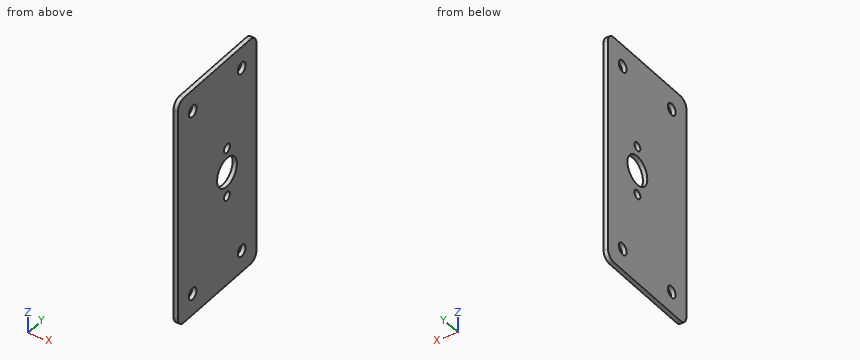
```python
from build123d import *

# Parameters (mm, degrees)
SKETCH_1_W      = 80
SKETCH_1_H      = 40
SKETCH_1_R      = 2
SKETCH_1_R_2    = 5.05
SKETCH_1_R_3    = 1.5
EXTRUDE_1_DEPTH = 1.5
FILLET_1_R      = 3


with BuildPart() as part:
    # ｽｹｯﾁ1 → ﾎﾞｽ - 押し出し1 (new body)
    with BuildSketch(Plane(origin=(0, 0, 0), x_dir=(0, 0, -1), z_dir=(1, 0, 0))):
        Rectangle(SKETCH_1_W, SKETCH_1_H)
        with Locations((32.5, 12.5)):
            Circle(SKETCH_1_R, mode=Mode.SUBTRACT)
        with Locations(Location((-32.5, 12.5, 0), (0, 0, 180))):
            Circle(SKETCH_1_R, mode=Mode.SUBTRACT)
        with Locations((32.5, -12.5)):
            Circle(SKETCH_1_R, mode=Mode.SUBTRACT)
        with Locations((0, 5)):
            Circle(SKETCH_1_R_2, mode=Mode.SUBTRACT)
        with Locations(Location((-32.5, -12.5, 0), (0, 0, 180))):
            Circle(SKETCH_1_R, mode=Mode.SUBTRACT)
        with Locations((8.5, 5)):
            Circle(SKETCH_1_R_3, mode=Mode.SUBTRACT)
        with Locations(Location((-8.5, 5, 0), (0, 0, 180))):
            Circle(SKETCH_1_R_3, mode=Mode.SUBTRACT)
    extrude(amount=EXTRUDE_1_DEPTH)

    # ﾌｨﾚｯﾄ1
    fillet_1_edges = [part.edges().sort_by_distance(p)[0] for p in [
        (0.75, -20, -40),
        (0.75, -20, 40),
        (0.75, 20, 40),
        (0.75, 20, -40),
    ]]
    fillet(fillet_1_edges, radius=FILLET_1_R)


solid = part.part
```
Could you check a few things on this model? Use its own coordinates, in mm. Give positions to 0.01 mm unless a question says otherwise; leave off trailing zeros. Loops run counter-clockwise (first coordinate to the right, second up) from the corner with the lowest first, then second, coordinate; pieces in that order, holes last. Notation, with made-up numbers: (-7, 26.5) -> (13, 26.5) arc R30 cw to (13, 65.5) -> close; hole circle Ø8 at (16, -18.75). An arc over 180 degrees is marked (long way). Put each result on its own line as item: value.
(1) Imagine slicing it at C-C on y = 5. Write out the boundary of the cut face in (x, z).
Computed:
outline: (0, -40) -> (1.5, -40) -> (1.5, -10) -> (0, -10) -> close; (0, -7) -> (1.5, -7) -> (1.5, -5.05) -> (0, -5.05) -> close; (0, 5.05) -> (1.5, 5.05) -> (1.5, 7) -> (0, 7) -> close; (0, 10) -> (1.5, 10) -> (1.5, 40) -> (0, 40) -> close
(2) Please list where these lines run through material, in increasing order: probe 1 along Y at (x, z) = (0.65, -32.5); probe 2 along Y at (x, z) = (0.3, -33.5); probe 3 along Z at (x, y) = (0.9, 11.5). Write a range as [from, to].
Computed:
probe 1: [-20, -14.5], [-10.5, 10.5], [14.5, 20]
probe 2: [-20, -14.23], [-10.77, 10.77], [14.23, 20]
probe 3: [-40, -34.23], [-30.77, 30.77], [34.23, 40]
(3) Imagine slicing it at A-A on z = 8.5. Write out the boundary of the cut face in (x, y).
Computed:
outline: (0, -20) -> (1.5, -20) -> (1.5, 3.5) -> (0, 3.5) -> close; (0, 6.5) -> (1.5, 6.5) -> (1.5, 20) -> (0, 20) -> close
(4) Imagine slicing it at B-B on z = 32.5. Write out the boundary of the cut face in (x, y).
Computed:
outline: (0, -20) -> (1.5, -20) -> (1.5, -14.5) -> (0, -14.5) -> close; (0, -10.5) -> (1.5, -10.5) -> (1.5, 10.5) -> (0, 10.5) -> close; (0, 14.5) -> (1.5, 14.5) -> (1.5, 20) -> (0, 20) -> close
(5) Imagine slicing it at D-D on y = -12.5. Write out the boundary of the cut face in (x, z).
Computed:
outline: (0, -40) -> (1.5, -40) -> (1.5, -34.5) -> (0, -34.5) -> close; (0, -30.5) -> (1.5, -30.5) -> (1.5, 30.5) -> (0, 30.5) -> close; (0, 34.5) -> (1.5, 34.5) -> (1.5, 40) -> (0, 40) -> close
